The model under review builds one solid part; all positions refer to its coordinate system, in mm. A direction names the side the tool comes from. Coordinates: 2 decimals unless noted, no trailing zeros. Order: outer loops, then holes, each group sorted by start corner. A loop starts at its lowest first (then second) coordinate and runs counter-clockwise, first axis right, second up. Notation, with made-up numbers: (-36.75, 87) - (11.25, 87) arc R20 cw to (11.25, 108) - close; hole circle Ø3 at (-34, 17). An arc over 180 degrees is marked (long way). Answer in a Markdown table with one row per item.
Autodesk Inventor part; units mm, degrees
ref_plane "YZ Plane" through (0, 0, 0) normal (1, 0, 0) x (0, 1, 0)
ref_plane "XZ Plane" through (0, 0, 0) normal (0, 1, 0) x (-1, 0, 0)
ref_plane "XY Plane" through (0, 0, 0) normal (0, 0, 1) x (1, 0, 0)
sketch "Sketch1" plane through (0, 0, 0) normal (0, 1, 0) x (-1, 0, 0)
  circle A0 centre (0, 0) radius 17
  dimension "d6" = 34
extrude "Extrusion1" add sketch "Sketch1" along normal blind 19.98
sketch "Sketch2" plane through (0, 19.98, 0) normal (0, 1, 0) x (1, 0, 0)
  circle A0 centre (0, 0) radius 15.5
  dimension "d9" = 31
extrude "Extrusion2" cut sketch "Sketch2" against normal blind 1.61
sketch "Sketch4" plane through (0, 0, 0) normal (0, -1, 0) x (1, 0, 0)
  circle A0 centre (0, 0) radius 15.5
  dimension "d15" = 31
extrude "Extrusion4" cut sketch "Sketch4" against normal blind 1.61
sketch "Sketch5" plane through (0, 0, 0) normal (0, -1, 0) x (1, 0, 0)
  circle A0 centre (0, 0) radius 17
  line L0 (17, 0) -> (17, 17)
  line L1 (17, 17) -> (17, 37)
  line L2 (17, 0) -> (17, -17)
  line L3 (17, -17) -> (17, -37)
  line L4 (17, 37) -> (37, 37)
  line L5 (37, 37) -> (37, -37)
  line L6 (37, -37) -> (17, -37)
  arc A1 (0, 17) -> (17, 37) centre (-9.2645, 42.0999) ccw
  circle A2 centre (0, 0) radius 14.285
  arc A3 (17, -37) -> (0, -17) centre (-9.2645, -42.0999) ccw
  point P0 (0, -17)
  dimension "d18" = 20
  dimension "d19" = 20
  dimension "d20" = 20
extrude "Extrusion5" add sketch "Sketch5" against normal blind 19.98 contours L2 L3 A3 A0 | A0 A1 L1 L0 | L0 L1 L4 L5 L6 L3 L2
sketch "Sketch7" plane through (0, 19.98, 0) normal (0, 1, 0) x (1, 0, 0)
  arc A0 (0, 17) -> (17, 37) centre (-9.2645, 42.0999) ccw
  line L0 (37, -37) -> (37, 37)
  line L1 (17, 37) -> (37, 37)
  line L2 (37, 37) -> (37, -37)
  line L3 (37, -37) -> (17, -37)
  line L4 (17, -37) -> (17, 37)
  point P0 (0, 0)
extrude "Extrusion6" add sketch "Sketch7" along normal blind 3
sketch "Sketch9" plane through (0, 0, 0) normal (0, -1, 0) x (1, 0, 0)
  line L0 (17, 37) -> (37, 37)
  line L1 (17, -37) -> (17, 37)
  line L2 (37, 37) -> (17, 37)
  line L3 (17, 37) -> (17, -37)
  line L4 (17, -37) -> (37, -37)
  line L5 (37, -37) -> (37, 37)
  point P0 (0, 0)
extrude "Extrusion7" add sketch "Sketch9" along normal blind 3
sketch "Sketch11" plane through (37, 22.98, 37) normal (1, 0, 0) x (0, 0, -1)
  line L0 (0, -3) -> (0, 0)
  line L1 (74, -22.98) -> (74, -25.98)
  line L2 (0, 0) -> (74, 0)
  line L3 (74, 0) -> (74, -25.98)
  line L4 (74, -25.98) -> (0, -25.98)
  line L5 (0, -25.98) -> (0, 0)
  point P0 (37, -22.98)
extrude "Extrusion8" add sketch "Sketch11" along normal blind 3
sketch "Sketch12" plane through (17, 19.98, 37) normal (0, 0, 1) x (1, 0, 0)
  line L0 (23, -22.98) -> (23, 3)
  line L1 (23, 0) -> (3, 0)
  line L2 (3, 0) -> (3, -19.98)
  line L3 (3, -19.98) -> (23, -19.98)
  line L4 (23, -19.98) -> (23, 0)
  line L5 (0, 3) -> (23, 3)
  line L6 (0, -19.98) -> (0, 0)
  line L7 (0, -22.98) -> (23, -22.98)
  point P0 (-17, -19.98)
  point P1 (23, -19.98)
  dimension "d29" = 3
  dimension "d30" = 3
  dimension "d31" = 3
extrude "Extrusion9" cut sketch "Sketch12" against normal through all
sketch "Sketch13" plane through (0, 18.37, 0) normal (0, 1, 0) x (1, 0, 0)
  line L0 (0, 7.29) -> (6.3133, 3.645)
  line L1 (6.3133, 3.645) -> (6.3133, -3.645)
  line L2 (6.3133, -3.645) -> (0, -7.29)
  line L3 (0, -7.29) -> (-6.3133, -3.645)
  line L4 (-6.3133, -3.645) -> (-6.3133, 3.645)
  line L5 (-6.3133, 3.645) -> (0, 7.29)
  point P0 (0, 0)
  point P1 (0, 0)
extrude "Extrusion10" cut sketch "Sketch13" against normal through all
sketch "Sketch14" plane through (0, 22.98, 0) normal (0, 1, 0) x (1, 0, 0)
  line L0 (40, 37) -> (40, -37)
  line L1 (17, -37) -> (40, -37)
  point P0 (0, 0)
  point P1 (28.5, 0)
  dimension "d37" = 11.5
  dimension "d38" = 37
hole "Hole1" at (28.5, 22.98, 0) direction (0, -1, 0) diameter 5.5 end through all
sketch "Sketch15" plane through (0, 22.98, 0) normal (0, 1, 0) x (1, 0, 0)
  circle A0 centre (28.5, -18.5) radius 3.0917
  circle A1 centre (28.5, 18.5) radius 2.226
  line L0 (17, 37) -> (40, 37)
  line L1 (17, -37) -> (40, -37)
  point P0 (0, 0)
  point P1 (28.5, 37)
  dimension "d47" = 18.5
  dimension "d48" = 18.5
hole "Hole2" at (28.5, 22.98, 18.5) at (28.5, 22.98, -18.5) direction (0, -1, 0) diameter 5.5 end through all
properties part number "CH-1-01-BearingBracket"
Item 1: We need section D-D, the plane y = 3.25. Write out the cut boundary in (x, z) (3 decimals), then the cut area to 3 significant figures.
Check values:
| item | result |
|---|---|
| outline | (0, -17) arc R26.755 cw to (17, -37) - (20, -37) - (20, 37) - (17, 37) arc R26.755 cw to (0, 17) arc R17 ccw to start; hole (-6.313, -3.645) - (0, -7.29) - (6.313, -3.645) - (6.313, 3.645) - (0, 7.29) - (-6.313, 3.645) - close |
| area | 1,330 mm^2 |
Item 2: We need section A-A, the plane x = 34.5. Write out the cut boundary in (y, z).
Check values:
| item | result |
|---|---|
| outline | (-3, -37) - (0, -37) - (0, 37) - (-3, 37) - close; (19.98, -37) - (22.98, -37) - (22.98, 37) - (19.98, 37) - close |
Item 3: We need section B-B, the plane x = 28.5. State how many separate pieces and enclosed holes the cut face has, then the cut area to 3 significant figures.
Check values:
| item | result |
|---|---|
| separate pieces | 8 |
| enclosed holes | 0 |
| area | 345 mm^2 |
Item 4: Clearance check with flat-ended pins moving along their axes: pin 1 Ø3.5 at (x, z) = (28.5, 0) entering from +Y; pin 2 Ø15.5 at (x, z) = (1, 0) entering from -Y; pin 3 Ø5 at (x, y) = (8.5, 2.5) entering from +Z; pin 4 Ø2 at (y, z) = (18.5, 21) entering from +X. State where each tip first meets the part, or that it passes through.
Check values:
| item | result |
|---|---|
| pin 1 | through |
| pin 2 | y = 1.61 |
| pin 3 | z = 24.63 |
| pin 4 | x = 20 |
Item 5: To check wall thickness, follow line 1 (Z direction, x = 28.5, y = -1); line 2 (X direction, y = 20.9, z = 18.5); line 3 (X direction, y = 18.85, z = 0). State the ranges of each line that lie inside material, in increasing order. Write a range as from..to.
Check values:
| item | result |
|---|---|
| line 1 | -37..-21.25, -15.75..-2.75, 2.75..15.75, 21.25..37 |
| line 2 | 17..25.75, 31.25..40 |
| line 3 | -17..-15.5, 15.5..20 |
Item 6: Tool access review of faces 4 (the face through (3.201, 10.107, 5.442)), 5 (the face through (20, 10, 1)), 6 (the face through (16, 19.98, 0)), 7 (the face through (7, 18.37, 0)), 8 (the face through (-2.018, 0.794, 15.368)): name each direction out of +Z, -Z, +X, -X, +Y, -Y from which nothing blocks a thin tool from reaching the whole face with its end or side.
Check values:
| item | result |
|---|---|
| face 4 | +Y, -Y |
| face 5 | +Z, -Z, +X |
| face 6 | +Z, -Z, -X, +Y |
| face 7 | +Y |
| face 8 | -Y |
Item 7: Mouldability with a two-part tool opening along Z and no side actions: class faces 1 (the face through (11, 9.85, 24.63)), 2 (the face through (32, 19.98, 1)), 3 (the face through (25.773, 21.459, 18.142)) as +Z half, -Z half, draft (parallel to the pull), parting line (faces both ways), or undercut.
Check values:
| item | result |
|---|---|
| face 1 | +Z half |
| face 2 | draft |
| face 3 | undercut |
